Autodesk Fusion 360 part; units mm, degrees
sketch "草图1" plane through (0, 0, 0) normal (0, 0, 1) x (1, 0, 0)
  line L0 (110, -137.5) -> (-110, -137.5)
  line L1 (-110, -137.5) -> (-110, 137.5)
  line L2 (-110, 137.5) -> (110, 137.5)
  line L3 (110, 137.5) -> (110, -137.5)
  line L4 (110, -137.5) -> (-110, 137.5) construction
  line L5 (-110, -137.5) -> (110, 137.5) construction
  line L6 (130, -157.5) -> (-130, -157.5)
  line L7 (-130, -157.5) -> (-130, 157.5)
  line L8 (-130, 157.5) -> (130, 157.5)
  line L9 (130, 157.5) -> (130, -157.5)
  line L10 (130, -157.5) -> (-130, 157.5) construction
  line L11 (-130, -157.5) -> (130, 157.5) construction
  line L12 (110, 137.5) -> (225, 137.5)
  line L13 (225, 137.5) -> (-225, 137.5)
  line L14 (0, 0) -> (0, 157.5) construction
  line L15 (0, 0) -> (0, -157.5) construction
  line L16 (-110, 137.5) -> (-110, 250)
  line L17 (-110, 250) -> (-110, -250)
  line L18 (0, 0) -> (-130, 0) construction
  line L19 (-225, 250) -> (225, 250)
  line L20 (225, 250) -> (225, -250)
  line L21 (225, -250) -> (-225, -250)
  line L22 (-225, -250) -> (-225, 250)
  line L23 (-225, 250) -> (225, -250) construction
  line L24 (225, 250) -> (-225, -250) construction
  line L25 (-130, 250) -> (-130, -250)
  line L26 (225, -157.5) -> (-225, -157.5)
  line L27 (-225, -137.5) -> (225, -137.5)
  line L28 (110, 250) -> (110, -250)
  line L29 (130, -250) -> (130, 250)
  line L30 (225, 157.5) -> (-225, 157.5)
  point P0 (-110, 0)
  dimension "d1" = 220
  dimension "d2" = 275
  dimension "d3" = 20
  dimension "d4" = 20
  dimension "d5" = 450
  dimension "d6" = 95
  dimension "d7" = 95
  dimension "d8" = 500
  dimension "d9" = 92.5
  dimension "d15" = 450
  dimension "d16" = 500
extrude "拉伸1" add sketch "草图1" along normal blind 20 contours L3 L9 L12 L13 L27 L28 L29 | L6 L9 L26 L27 L28 L29 | L1 L7 L13 L17 L25 L27 | L6 L7 L17 L25 L26 L27 | L8 L9 L12 L13 L28 L29 L30 | L6 L21 L26 L28 L29 | L7 L8 L13 L16 L17 L25 L30 | L6 L17 L21 L25 L26 | L8 L19 L28 L29 L30 | L8 L16 L17 L19 L25 L30 makes body 1 at (-110, 83.3333, 6.6667) makes body 2 at (130, 83.3333, 6.6667)
extrude "拉伸2" add sketch "草图1" against normal blind 20 contours L0 L6 L17 L26 L27 L28 | L6 L9 L26 L27 L28 L29 | L6 L7 L17 L25 L26 L27 | L8 L9 L12 L13 L28 L29 L30 | L2 L8 L13 L16 L17 L28 L30 | L9 L20 L26 L27 L29 | L7 L8 L13 L16 L17 L25 L30 | L7 L22 L25 L26 L27 | L9 L12 L13 L20 L29 L30 | L7 L13 L22 L25 L30 bodies 1 2
chamfer "倒角1" distance 20 angle 45 8 edges at (-120, -157.5, 0) (120, -157.5, 0) (-120, 137.5, 0) (120, 137.5, 0) (-120, -137.5, 0) (-120, 157.5, 0) (120, 157.5, 0) (120, -137.5, 0) on bodies 1
sketch "草图2" plane through (0, 0, -20) normal (0, 0, -1) x (1, 0, 0)
  line L0 (-225, 157.5) -> (-225, 137.5)
  line L1 (-225, 137.5) -> (-130, 137.5)
  line L2 (-130, 137.5) -> (-110, 137.5)
  line L3 (-110, 137.5) -> (110, 137.5)
  line L4 (110, 137.5) -> (130, 137.5)
  line L5 (130, 137.5) -> (225, 137.5)
  line L6 (225, 137.5) -> (225, 157.5)
  line L7 (225, 157.5) -> (130, 157.5)
  line L8 (130, 157.5) -> (110, 157.5)
  line L9 (110, 157.5) -> (-110, 157.5)
  line L10 (-110, 157.5) -> (-130, 157.5)
  line L11 (-130, 157.5) -> (-225, 157.5)
  line L12 (-130, 157.5) -> (-130, 137.5) construction
  line L13 (-110, 157.5) -> (-110, 137.5) construction
  line L14 (110, 157.5) -> (110, 137.5) construction
  line L15 (130, 157.5) -> (130, 137.5) construction
  line L16 (-225, 147.5) -> (225, 147.5) construction
  circle A0 centre (-185.15, 147.5) radius 2.65
  circle A1 centre (-164.85, 147.5) radius 2.65
  circle A2 centre (164.85, 147.5) radius 2.65
  circle A3 centre (185.15, 147.5) radius 2.65
  circle A4 centre (-75.15, 147.5) radius 2.65
  circle A5 centre (-54.85, 147.5) radius 2.65
  circle A6 centre (54.85, 147.5) radius 2.65
  circle A7 centre (75.15, 147.5) radius 2.65
  point P0 (-185.15, 147.5)
  point P1 (-164.85, 147.5)
  point P2 (164.85, 147.5)
  point P3 (185.15, 147.5)
  point P4 (-75.15, 147.5)
  point P5 (-54.85, 147.5)
  point P6 (75.15, 147.5)
  point P7 (54.85, 147.5)
  dimension "d17" = 55.15
  dimension "d18" = 55.15
  dimension "d19" = 20.3
  dimension "d20" = 20.3
  dimension "d21" = 5.3
  dimension "d22" = 5.3
  dimension "d23" = 5.3
  dimension "d24" = 5.3
  dimension "d25" = 55.15
  dimension "d26" = 55.15
  dimension "d27" = 20.3
  dimension "d28" = 20.3
  dimension "d29" = 5.3
  dimension "d30" = 5.3
  dimension "d31" = 5.3
  dimension "d32" = 5.3
extrude "拉伸3" cut sketch "草图2" against normal blind 10 contours A0 | A1 | A2 | A3 | A4 | A5 | A6 | A7 bodies 1
sketch "草图3" plane through (0, 0, -20) normal (0, 0, -1) x (1, 0, 0)
  line L0 (225, -157.5) -> (225, -137.5)
  line L1 (225, -137.5) -> (130, -137.5)
  line L2 (130, -137.5) -> (110, -137.5)
  line L3 (110, -137.5) -> (-110, -137.5)
  line L4 (-110, -137.5) -> (-130, -137.5)
  line L5 (-130, -137.5) -> (-225, -137.5)
  line L6 (-225, -137.5) -> (-225, -157.5)
  line L7 (-225, -157.5) -> (-130, -157.5)
  line L8 (-130, -157.5) -> (-110, -157.5)
  line L9 (-110, -157.5) -> (110, -157.5)
  line L10 (110, -157.5) -> (130, -157.5)
  line L11 (130, -157.5) -> (225, -157.5)
  line L12 (-130, -137.5) -> (-130, -157.5)
  line L13 (-110, -137.5) -> (-110, -157.5)
  line L14 (110, -137.5) -> (110, -157.5)
  line L15 (130, -137.5) -> (130, -157.5)
  line L16 (225, -147.5) -> (-225, -147.5) construction
  circle A0 centre (-185.15, -147.5) radius 2.65
  circle A1 centre (-164.85, -147.5) radius 2.65
  circle A2 centre (-75.15, -147.5) radius 2.65
  circle A3 centre (-54.85, -147.5) radius 2.65
  circle A4 centre (54.85, -147.5) radius 2.65
  circle A5 centre (75.15, -147.5) radius 2.65
  circle A6 centre (164.85, -147.5) radius 2.65
  circle A7 centre (185.15, -147.5) radius 2.65
  point P0 (-164.85, -147.5)
  point P1 (-185.15, -147.5)
  point P2 (-75.15, -147.5)
  point P3 (-54.85, -147.5)
  point P4 (54.85, -147.5)
  point P5 (75.15, -147.5)
  point P6 (164.85, -147.5)
  point P7 (185.15, -147.5)
  dimension "d35" = 5.3
  dimension "d36" = 5.3
  dimension "d37" = 5.3
  dimension "d38" = 5.3
  dimension "d39" = 5.3
  dimension "d40" = 5.3
  dimension "d41" = 5.3
  dimension "d42" = 5.3
  dimension "d43" = 55.15
  dimension "d44" = 55.15
  dimension "d45" = 55.15
  dimension "d46" = 55.15
  dimension "d47" = 20.3
  dimension "d48" = 20.3
  dimension "d49" = 20.3
  dimension "d50" = 20.3
extrude "拉伸4" cut sketch "草图2" sketch "草图3" against normal blind 5 contours A0 | A1 | A2 | A3 | A4 | A5 | A6 | A7 of sketch 2 contours A0 | A1 | A2 | A3 | A4 | A5 | A6 | A7 bodies 1
Verification items for the finished model (mm, model axes). A direction names the side the tool comes from. Give positions to 0.01 mm unless a question says otherwise; leave off trailing zeros. Write each loop counter-clockwise with the first axis right and the second up, starting at its lowest first coordinate (ties: lowest second). Pieces come first, ordered by that corner, then holes. Notation, with made-up numbers: M 22.25,68 L 34.25,68 A22 ccw 34.25,78 Z; hole C -36,89.25 d7. An arc over 180 degrees is marked long. Put each result on its own line as item: value. Start each with the question number.
1. Go/stop test with flat-tipped pins: pin 1 Ø1.6 at (x, y) = (-184.5, -148) entering from -Z; pin 2 Ø8.5 at (x, y) = (54.85, -147.5) entering from +Z; pin 3 Ø6 at (y, z) = (-188, 10) entering from -X; pin 4 Ø7 at (x, y) = (-164.85, 147.5) entering from -Z. Record where each tip stops, or that it passes through.
2. Section check B-B (x = 11). Record the cut outline in (y, z), and give its area (3 significant figures).
3. Scan lines: line 1 along Y through (x, z) = (-185.15, -18.5); line 2 along X through (y, z) = (0.5, 4); line 3 along Y through (x, z) = (1.5, -15). Record each from-to range of solid material in increasing order. Write a range as [from, to].
4. Section check A-A (y = -110.5). Record the cut outline in (x, z).
5. Set-up check for faces 4 (the face through (120, -213, 0)), 5 (the face through (-2, 148, 0)), 6 (the face through (-178, -147, 0)), 7 (the face through (-119.86, 127.642, -10.138)): record each of +Z, -Z, +X, -X, +Y, -Y from which the full face is reachable in a straight line by a thin tool's end or side.
6. Draft check along X on faces 1 (the face through (-3, -147, -20)), 2 (the face through (-225, -148, -10)), 3 (the face through (-110, -3, 9)). Enter one of: +X half, -X half, draft (parallel to the pull), parting line (faces both ways), or undercut.
Answer list:
1. pin 1: z = -10
1. pin 2: z = 0
1. pin 3: x = -130
1. pin 4: z = -20
2. outline: M -157.5,-20 L -137.5,-20 L -137.5,0 L -157.5,0 Z; M 137.5,-20 L 157.5,-20 L 157.5,0 L 137.5,0 Z
2. area: 800 mm2
3. line 1: [-157.5, -150.15], [-144.85, -137.5], [137.5, 144.85], [150.15, 157.5]
3. line 2: [-130, -110], [110, 130]
3. line 3: [-157.5, -137.5], [137.5, 157.5]
4. outline: M -130,0 L -110,0 L -110,20 L -130,20 Z; M 110,0 L 130,0 L 130,20 L 110,20 Z
5. face 4: -Z, +X, -X, -Y
5. face 5: +Z, +Y, -Y
5. face 6: +Z, -X, +Y, -Y
5. face 7: -Z, +X, -X
6. face 1: draft
6. face 2: -X half
6. face 3: undercut
